Input: part model. Units: mm. Frame: model coordinates. Coordinates: 2 decimals unless noted, no trailing zeros. Use one line per item in the form item = value.
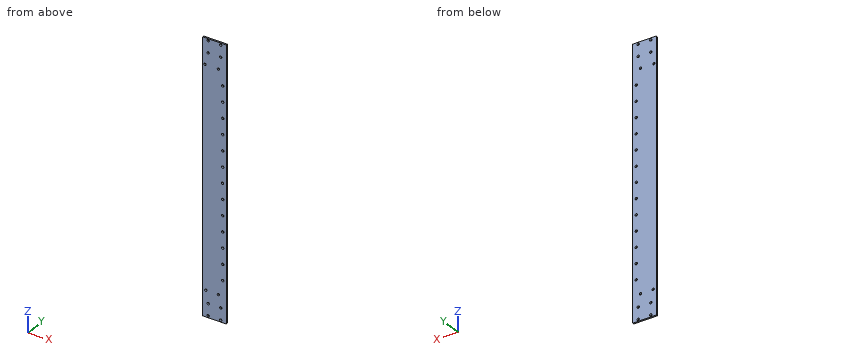
from build123d import *

# Parameters (mm, degrees)
BOSS_EXTRUDE1_DEPTH      = 200
BOSS_EXTRUDE1_DEPTH_BACK = 144
SKETCH1_W                = 30
SKETCH1_H                = 2
F_3_0_3_DIAMETER_SLOT1_D = 3
F_3_0MM_DOWEL_HOLE1_D    = 3


with BuildPart() as part:
    # Sketch1 → Boss-Extrude1 (new, two sides: drawn at the far end of the back side and taken through both)
    with BuildSketch(Plane.XY.offset(-BOSS_EXTRUDE1_DEPTH_BACK)):
        Rectangle(SKETCH1_W, SKETCH1_H)
    extrude(amount=BOSS_EXTRUDE1_DEPTH + BOSS_EXTRUDE1_DEPTH_BACK)

    # Ø3.0 (3) Diameter Slot1 (through all)
    with Locations(Plane(origin=(0, 1, 0), x_dir=(1, 0, 0), z_dir=(0, 1, 0))):
        with Locations((-8.05, 126.5), (7.95, 126.5), (7.95, 141.5), (-8.05, 141.5)):
            Hole(F_3_0_3_DIAMETER_SLOT1_D / 2)

    # Ø3.0mm Dowel Hole1 (through all)
    with Locations(Plane(origin=(0, -1, 0), x_dir=(-1, 0, 0), z_dir=(0, -1, 0))):
        with Locations((-7.95, -197.5), (8.05, -197.5), (8.05, -182.5), (-7.95, -182.5), (-5, -167), (12, -167), (-10.5, -148), (-10.5, -128), (-10.5, -108), (-10.5, -88), (-10.5, -68), (-10.5, -48), (-10.3, -28), (-10.5, -8), (-10.5, 12), (-10.5, 32), (-10.5, 52), (-10.5, 72), (-10.5, 92), (-5, 111), (11, 111)):
            Hole(F_3_0MM_DOWEL_HOLE1_D / 2)


solid = part.part
(1) Section query A-A on y = -0.05. State how many separate pieces and enclosed holes the cut face has, plus the area to 3 significant figures.
Computed:
separate_pieces = 1
enclosed_holes = 25
area = 10,100 mm^2
(2) Line query: probe 1 along Z at (x, y) = (8, 0.35); probe 2 along X at (y, z) = (0.15, 167); probe 3 along X at (y, z) = (-0.3, -126.5). Output: solid intervals per line, ascending.
Computed:
probe_1 = -144 to -143, -140 to -128, -125 to 181, 184 to 196, 199 to 200
probe_2 = -15 to -13.5, -10.5 to 3.5, 6.5 to 15
probe_3 = -15 to -9.55, -6.55 to 6.45, 9.45 to 15
(3) First-contact query: pin 1 Ø3.5 at (x, z) = (-11, -111) entering from +Y; pin 2 Ø2.5 at (x, z) = (10.5, 48) entering from -Y. Flat tips, straight axial feed; report the tip coordinate or a pass-through.
Computed:
pin_1 = 1
pin_2 = through
